The model under review builds one solid part; all positions refer to its coordinate system, in mm. A direction names the side the tool comes from. Give positions to 0.01 mm unless a question says otherwise; leave off trailing zeros. Order: outer loops, then holes, each group sorted by start corner. A loop starts at its lowest first (then second) coordinate and runs counter-clockwise, first axis right, second up. Notation, with made-up numbers: (85.25, -24) - (98.25, -24) arc R21 ccw to (98.25, -2) - close; hole circle Ø6 at (44.25, 23.25). An arc over 180 degrees is marked (long way). Write item = value, one per line. Start each with the question number.
1. Mouldability with a two-part tool opening along Y and no side actions: class faces 4 (the cylindrical face through (-23.3, -11.5, 24.6)), 5 (the flat face through (-15, -12, 25)), 6 (the flat face through (-27.37, -2.65, 24.65)) as pulls with the +Y half, pulls with the -Y half, needs draft (parallel to the pull), parting line crosses it, or undercut.
2. Machinability: for faces 1 (the flat face through (27.37, -2.65, 24.65)), 2 (the flat face through (-27.582, -7.196, 24.65)), 3 (the flat face through (-25.556, -17.693, 24.65)), which of the approach directions +Z, -Z, +X, -X, +Y, -Y give a long, thin tool a straight path to every point of the face, cutting with its end or side? Answer none if there is none.
3. We need section A-A, the plane y = -9.75. Give the boundary of the cut face in (x, z), and give its area (3 significant figures).
4. Wall thickness on probe 1 along X at (y, z) = (-8.25, 43.5); probe 2 along X at (y, z) = (-14.5, 12.5); probe 3 along Y at (x, z) = (3.5, 45): over which ranges is each line inside the solid? List them lowest first.
5. We need section B-B, the plane x = 9. Give the boundary of the cut face in (y, z).
6. For P1, Ø10, axis at x = -23.5, y = -12.5, coming from the -Z side; P2, Ø5, axis at y = -13.5, z = 31.5, coming from the +X side; P3, Ø1, axis at y = -11.5, z = 8, coming from the -X side; P4, Ø1, axis at x = 9, z = 41.5, coming from the -Y side, all flat-tipped, find the tip position at first contact; note any pin that passes through.
from build123d import *

# Parameters (mm, degrees)
PAD_DEPTH = 50


with BuildPart() as part:
    # Sketch → Pad (new body)
    with BuildSketch(Plane.XY):
        with BuildLine():
            Line((0, 0), (0, -4))
            Line((0, -4), (-15, -4))
            Line((-15, -4), (-15, -20))
            Line((-15, -20), (-15.962702, -20))
            ThreePointArc((-16.758832, -19.235543), (-16.514566, -19.777943), (-15.962702, -20))
            Line((-16.758832, -19.235543), (-17.191233, -8.587361))
            ThreePointArc((-17.191233, -8.587361), (-18.663554, -7.148457), (-20.185686, -8.534564))
            Line((-21.030971, -19.657951), (-20.185686, -8.534564))
            ThreePointArc((-21.76856, -19.663558), (-21.397187, -19.999989), (-21.030971, -19.657951))
            Line((-21.76856, -19.663558), (-22.443519, -12.270938))
            ThreePointArc((-22.443519, -12.270938), (-23.300533, -11.498289), (-24.138133, -12.291944))
            Line((-24.626417, -19.650386), (-24.138133, -12.291944))
            ThreePointArc((-25.372798, -19.660239), (-24.995058, -19.999967), (-24.626417, -19.650386))
            Line((-25.372798, -19.660239), (-25.743648, -15.669538))
            ThreePointArc((-25.743648, -15.669538), (-26.587631, -14.898227), (-27.435897, -15.664825))
            Line((-27.830084, -19.664747), (-27.435897, -15.664825))
            ThreePointArc((-28.571641, -19.621239), (-28.221771, -19.999362), (-27.830084, -19.664747))
            Line((-28.571641, -19.621239), (-28.540106, -17.959608))
            ThreePointArc((-28.540106, -17.959608), (-28.907829, -17.394963), (-29.568372, -17.528109))
            Line((-31.830105, -19.834306), (-29.568372, -17.528109))
            ThreePointArc((-32.435415, -19.2943), (-32.390304, -19.852993), (-31.830105, -19.834306))
            Line((-32.435415, -19.2943), (-29.926108, -16.198984))
            ThreePointArc((-29.926108, -16.198984), (-29.834934, -15.3395), (-30.578403, -14.898728))
            Line((-32.030902, -14.952159), (-30.578403, -14.898728))
            ThreePointArc((-32.071041, -14.048146), (-32.499555, -14.52007), (-32.030902, -14.952159))
            Line((-32.071041, -14.048146), (-28.20584, -13.847076))
            ThreePointArc((-28.20584, -13.847076), (-27.40004, -13.006636), (-28.189047, -12.150411))
            Line((-32.160387, -11.864905), (-28.189047, -12.150411))
            ThreePointArc((-32.153271, -11.134653), (-32.499983, -11.496435), (-32.160387, -11.864905))
            Line((-32.153271, -11.134653), (-25.697743, -10.796857))
            ThreePointArc((-25.697743, -10.796857), (-24.750068, -9.810055), (-25.674128, -8.801106))
            Line((-32.119375, -8.310687), (-25.674128, -8.801106))
            ThreePointArc((-32.114723, -7.488986), (-32.499993, -7.897668), (-32.119375, -8.310687))
            Line((-32.114723, -7.488986), (-22.920848, -6.894049))
            ThreePointArc((-22.920848, -6.894049), (-21.050015, -4.89004), (-22.937185, -2.901408))
            Line((-31.68374, -2.407258), (-22.937185, -2.901408))
            ThreePointArc((-32.5, -1.543581), (-32.263646, -2.137765), (-31.68374, -2.407258))
            Line((-32.5, -1.543581), (-32.5, -0.517038))
            ThreePointArc((-31.982962, 0), (-32.348563, -0.151437), (-32.5, -0.517038))
            Line((-31.982962, 0), (0, 0))
        make_face()
    pad = extrude(amount=PAD_DEPTH)

    # Mirrored: Pad across Sketch V_Axis
    add(pad.mirror(Plane(origin=(0, 0, 0), x_dir=(0, 0, 1), z_dir=(1, 0, 0))))


solid = part.part
Model answer:
q1.face_4 = pulls with the -Y half
q1.face_5 = needs draft
q1.face_6 = undercut
q2.face_1 = +Z, -Z, +X
q2.face_2 = +Z, -Z, -X
q2.face_3 = +Z, -Z, -Y
q3.outline = (-24.75, 0) - (-20.28, 0) - (-20.28, 50) - (-24.75, 50) - close; (-17.14, 0) - (-15, 0) - (-15, 50) - (-17.14, 50) - close; (15, 0) - (17.14, 0) - (17.14, 50) - (15, 50) - close; (20.28, 0) - (24.75, 0) - (24.75, 50) - (20.28, 50) - close
q3.area = 662 mm2
q4.probe_1 = -32.31 to -20.14, -17.24 to -15, 15 to 17.24, 20.14 to 32.31
q4.probe_2 = -32.5 to -24.28, -22.24 to -20.64, -16.95 to -15, 15 to 16.95, 20.64 to 22.24, 24.28 to 32.5
q4.probe_3 = -4 to 0
q5.outline = (-4, 0) - (0, 0) - (0, 50) - (-4, 50) - close
q6.P1 = 0
q6.P2 = 32.5
q6.P3 = -32.5
q6.P4 = -4
